Geometry check sheet. Reference: the model listing, model coordinates, mm. Face numbers are marked on the shaded views. A direction names the side the tool comes from. Give positions to 0.01 mm unless a question says otherwise; leave off trailing zeros. Loops run counter-clockwise (first coordinate to the right, second up) from the corner with the lowest first, then second, coordinate; pieces in that order, holes last. Notation, with made-up numbers: (-33, 79.25) -> (1, 79.25) arc R25 cw to (1, 113.25) -> close; hole circle Ø10 at (54.5, 43.25). An arc over 180 degrees is marked (long way). One line per item, written item: value. Start each with the question number.
(1) Gauge pin test, flat ends, axial feed: pin 1 Ø2 at (x, z) = (-6, 8.5) entering from -Y; pin 2 Ø3 at (y, z) = (-3, 9) entering from +X. Record the tip position at first contact, or that the pin passes through.
(2) Tool access check on the marked faces 1 and 2. Record the directions out of +Z, -Z, +X, -X, +Y, -Y that give a thin tool (end or side, any length) a straight path to the whole face; none if there is none.
(3) Sectioned sample at D-D, the plane y = -6.75. Record the cut outline in (x, z).
(4) Scan lines: line 1 along Y through (x, z) = (0, 5.5) (3 decimals); line 2 along Z through (x, y) = (-7.25, -1.5); line 3 along X through (y, z) = (-2.5, 1.5). Record each from-to range of solid material in increasing order. Write a range as from..to.
(5) Sectioned sample at C-C, the plane z = 4.25. Record the cut outline in (x, y) (3 decimals), then the cut area to 3 significant figures.
(6) Sectioned sample at B-B, the plane y = 2.75. Record the cut outline in (x, z), then the cut area to 3 significant figures.
(7) Draft check along Z on the marked faces 3, 4, 5 and 6. Enter one of: pulls with the +Z half, pulls with the -Z half, needs draft (parallel to the pull), parting line crosses it, or undercut.
(8) Sectioned sample at A-A, the plane x = 0. Record the cut outline in (y, z) (3 decimals).
from build123d import *

# Parameters (mm, degrees)
SKETCH1_R           = 9.525
BOSS_EXTRUDE1_DEPTH = 2.54
SKETCH2_R           = 6.35
BOSS_EXTRUDE2_DEPTH = 7.62
CUT_EXTRUDE1_REACH  = 14.7
SKETCH4_R           = 3.175


with BuildPart() as part:
    # Sketch1 → Boss-Extrude1 (new body)
    with BuildSketch(Plane.XY):
        Circle(SKETCH1_R)
    boss_extrude1 = extrude(amount=BOSS_EXTRUDE1_DEPTH)

    # Sketch2 → Boss-Extrude2 (add)
    with BuildSketch(Plane.XY.offset(2.54)):
        Circle(SKETCH2_R)
    extrude(amount=BOSS_EXTRUDE2_DEPTH)

    # Mirror1: Boss-Extrude1 across plane
    add(boss_extrude1.mirror(Plane.XY.offset(6.35)))

    # Sketch4 → Cut-Extrude1 (cut, up to next)
    with BuildSketch(Plane.XY.offset(12.7), mode=Mode.PRIVATE) as cut_extrude1_sk1:
        Circle(SKETCH4_R)
    cut_extrude1_tool1 = extrude(cut_extrude1_sk1.sketch, amount=-CUT_EXTRUDE1_REACH, mode=Mode.PRIVATE) & part.part
    add(cut_extrude1_tool1.solids().sort_by_distance((0, 0, 12.7))[0], mode=Mode.SUBTRACT)


solid = part.part
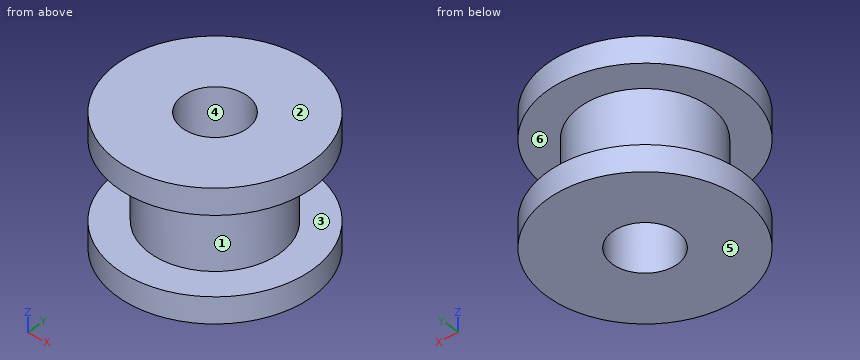
Calculated:
1. pin 1: stops at y = -3.91
1. pin 2: stops at x = 9.3
2. face 1: none
2. face 2: +Z, +X, -X, +Y, -Y
3. outline: (-6.72, 0) -> (6.72, 0) -> (6.72, 2.54) -> (-6.72, 2.54) -> close; (-6.72, 10.16) -> (6.72, 10.16) -> (6.72, 12.7) -> (-6.72, 12.7) -> close
4. line 1: y = -6.35..-3.175, 3.175..6.35
4. line 2: z = 0..2.54, 10.16..12.7
4. line 3: x = -9.19..-1.96, 1.96..9.19
5. outline: circle Ø12.7 at (0, 0); hole circle Ø6.35 at (0, 0)
5. area: 95.0 mm2
6. outline: (-9.12, 0) -> (-1.59, 0) -> (-1.59, 12.7) -> (-9.12, 12.7) -> (-9.12, 10.16) -> (-5.72, 10.16) -> (-5.72, 2.54) -> (-9.12, 2.54) -> close; (1.59, 0) -> (9.12, 0) -> (9.12, 2.54) -> (5.72, 2.54) -> (5.72, 10.16) -> (9.12, 10.16) -> (9.12, 12.7) -> (1.59, 12.7) -> close
6. area: 140 mm2
7. face 3: undercut
7. face 4: needs draft
7. face 5: pulls with the -Z half
7. face 6: undercut
8. outline: (-9.525, 0) -> (-3.175, 0) -> (-3.175, 12.7) -> (-9.525, 12.7) -> (-9.525, 10.16) -> (-6.35, 10.16) -> (-6.35, 2.54) -> (-9.525, 2.54) -> close; (3.175, 0) -> (9.525, 0) -> (9.525, 2.54) -> (6.35, 2.54) -> (6.35, 10.16) -> (9.525, 10.16) -> (9.525, 12.7) -> (3.175, 12.7) -> close
